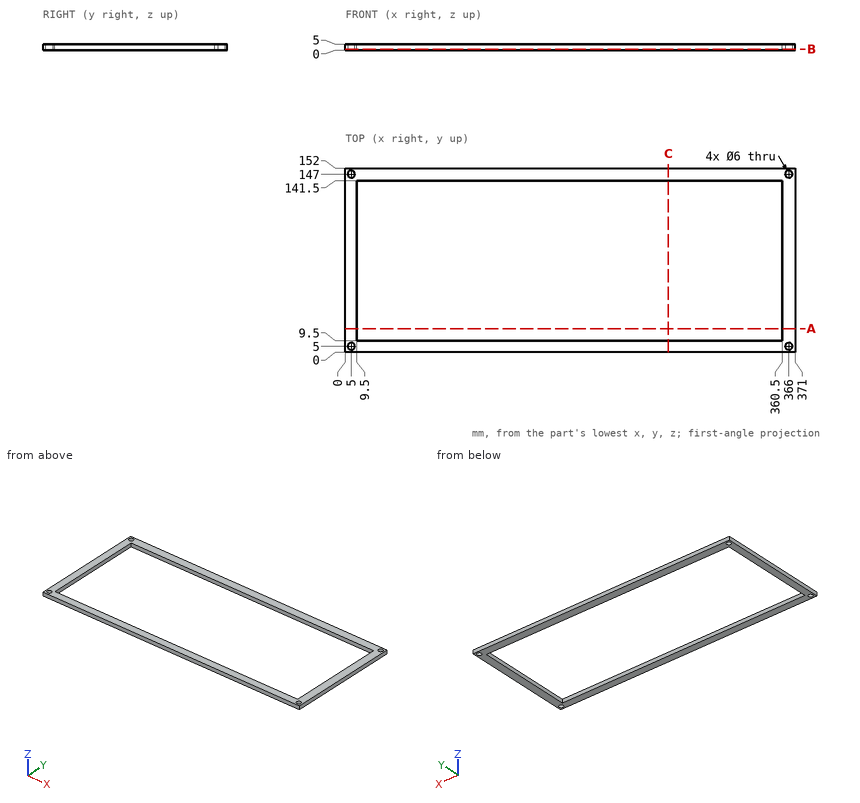
Geometry check sheet. Reference: drawing and pictorial views, mm from the part's lowest x, y, z. Round coordinates to 2 decimals unless told otherwise and drop trailing zeros. Loops run counter-clockwise (first coordinate to the right, second up) from the corner with the lowest first, then second, coordinate; pieces in that order, holes last. Notation, with made-up numbers: (-24, 79) - (-15, 79) arc R26 ccw to (-15, 94) - close; hole circle Ø2 at (56.25, 31). An arc over 180 degrees is marked (long way). One line per question, with ' | ' between items. Start each with the question number.
1. Cross-section at A-A on y = 19.5. Record the cut outline in (x, z), then the cut area to 3 significant figures.
2. Cross-section at C-C on x = 266.5. Record the cut outline in (y, z), then the cut area to 3 significant figures.
3. Cross-section at B-B on z = 0.75. Record the cut outline in (x, y).
4. Scan lines: line 1 (Y direction, x = 366, z = 1.8); line 2 (Y direction, x = 115, z = 2.2); line 3 (X direction, y = 19, z = 4.3). Record each from-to range of solid material in increasing order. Write a range as [from, to].
Taken from the geometry:
1) outline: (0, 0) - (9.5, 0) - (9.5, 5) - (0, 5) - close; (360.5, 0) - (371, 0) - (371, 5) - (360.5, 5) - close | area: 100 mm²
2) outline: (0, 0) - (9.5, 0) - (9.5, 5) - (0, 5) - close; (141.5, 0) - (152, 0) - (152, 5) - (141.5, 5) - close | area: 100 mm²
3) outline: (0, 0) - (371, 0) - (371, 152) - (0, 152) - close; hole circle Ø6 at (5, 5); hole circle Ø6 at (5, 147); hole (9.5, 9.5) - (360.5, 9.5) - (360.5, 141.5) - (9.5, 141.5) - close; hole circle Ø6 at (366, 5); hole circle Ø6 at (366, 147)
4) line 1: [0, 2], [8, 144], [150, 152] | line 2: [0, 9.5], [141.5, 152] | line 3: [0, 9.5], [360.5, 371]
